```python
from build123d import *
from build123d.topology import SkipClean

# Parameters (mm, degrees)
SKETCH1_W           = 52.3
SKETCH1_H           = 52.3
SKETCH1_R           = 11.5
SKETCH1_R_2         = 1.75
BOSS_EXTRUDE1_DEPTH = 3
SKETCH2_W           = 52.3
SKETCH2_H           = 5
BOSS_EXTRUDE2_DEPTH = 40
SKETCH3_W           = 3
SKETCH3_H           = 5
CUT_EXTRUDE1_DEPTH  = 71.845695
BOSS_EXTRUDE3_DEPTH = 4.9
FILLET1_R           = 5
FILLET2_R           = 2
SKETCH5_W           = 10
SKETCH5_H           = 7
SKETCH5_R           = 1.3
BOSS_EXTRUDE4_DEPTH = 5
SKETCH6_W           = 7
SKETCH6_H           = 10
SKETCH6_R           = 1.35
BOSS_EXTRUDE5_DEPTH = 5
FILLET3_R           = 3
FILLET4_R           = 3
SKETCH7_R           = 3.3734375
BOSS_EXTRUDE6_DEPTH = 25.4
FILLET5_R           = 2
CUT_EXTRUDE2_DEPTH  = 85.05422357
FILLET6_START       = -26.15
FILLET6_DEPTH       = 7.129662431
FILLET6_START_2     = -20.042964894
FILLET6_2_DEPTH     = 4.85752147
FILLET6_START_3     = -16.0065624
FILLET6_3_DEPTH     = 2.695573852
FILLET6_4_DEPTH     = 1.974476163
FILLET6_5_DEPTH     = 1.685079156
FILLET6_START_4     = 2.9999999
FILLET6_6_DEPTH     = 22.4000001
FILLET6_START_5     = 5.780256625
FILLET6_7_DEPTH     = 0.960746932


with BuildPart() as part:
    # Sketch1 → Boss-Extrude1 (new body)
    with BuildSketch(Plane.XY):
        Rectangle(SKETCH1_W, SKETCH1_H)
        Circle(SKETCH1_R, mode=Mode.SUBTRACT)
        with Locations((-15.5, 15.5)):
            Circle(SKETCH1_R_2, mode=Mode.SUBTRACT)
        with Locations((15.5, 15.5)):
            Circle(SKETCH1_R_2, mode=Mode.SUBTRACT)
        with Locations((-15.5, -15.5)):
            Circle(SKETCH1_R_2, mode=Mode.SUBTRACT)
        with Locations((15.5, -15.5)):
            Circle(SKETCH1_R_2, mode=Mode.SUBTRACT)
    extrude(amount=BOSS_EXTRUDE1_DEPTH)

    # Sketch2 → Boss-Extrude2 (add)
    with BuildSketch(Plane(origin=(0, 0, 0), x_dir=(-1, 0, 0), z_dir=(0, 0, -1))):
        with Locations((0, -23.65)):
            Rectangle(SKETCH2_W, SKETCH2_H)
    extrude(amount=BOSS_EXTRUDE2_DEPTH)

    # Sketch3 → Cut-Extrude1 (cut, through all)
    with BuildSketch(Plane(origin=(26.15, 0, 0), x_dir=(0, 0, -1), z_dir=(1, 0, 0))):
        with Locations((-1.5, 23.65)):
            Rectangle(SKETCH3_W, SKETCH3_H)
    extrude(amount=-CUT_EXTRUDE1_DEPTH, mode=Mode.SUBTRACT)

    # Sketch4 → Boss-Extrude3 (add)
    with BuildSketch(Plane(origin=(26.15, 0, 0), x_dir=(0, 0, -1), z_dir=(1, 0, 0))):
        Polygon((0, 16.15), (25, -21.15), (20.184652233, -21.15), (0, 8.965501131), align=None)
    boss_extrude3 = extrude(amount=-BOSS_EXTRUDE3_DEPTH)

    # Mirror1: Boss-Extrude3 across plane
    add(boss_extrude3.mirror(Plane(origin=(0, 0, 0), x_dir=(0, 0, 1), z_dir=(1, 0, 0))))

    # Fillet1
    fillet1_edges = [part.edges().sort_by_distance(p)[0] for p in [
        (-26.15, -23.65, -40),
        (26.15, -23.65, -40),
        (-26.15, 21.15, 1.5),
        (26.15, 21.15, 1.5),
    ]]
    fillet(fillet1_edges, radius=FILLET1_R)

    # Fillet2
    fillet2_edges = [part.edges().sort_by_distance(p)[0] for p in [
        (23.7, 8.965501131, 0),
        (23.7, 16.15, 0),
        (23.7, -21.15, -25),
        (23.7, -21.15, -20.184652233),
        (-23.7, 16.15, 0),
        (-23.7, 8.965501131, 0),
        (-23.7, -21.15, -20.184652233),
        (-23.7, -21.15, -25),
    ]]
    fillet(fillet2_edges, radius=FILLET2_R)

    # Sketch5 → Boss-Extrude4 (add)
    with BuildSketch(Plane(origin=(0, -26.15, 0), x_dir=(1, 0, 0), z_dir=(0, 1, 0))):
        with Locations((-31.15, 0.5)):
            Rectangle(SKETCH5_W, SKETCH5_H)
        with Locations((-32.15, 0.5)):
            Circle(SKETCH5_R, mode=Mode.SUBTRACT)
    boss_extrude4 = extrude(amount=BOSS_EXTRUDE4_DEPTH)

    # Mirror2: Boss-Extrude4 across plane
    add(boss_extrude4.mirror(Plane(origin=(0, 0, 0), x_dir=(0, 0, 1), z_dir=(1, 0, 0))))

    # Sketch6 → Boss-Extrude5 (add)
    with BuildSketch(Plane.XZ.offset(26.15)):
        with Locations((0, -45)):
            Rectangle(SKETCH6_W, SKETCH6_H)
        with Locations(Location((0, -46, 0), (0, 0, 270))):
            Circle(SKETCH6_R, mode=Mode.SUBTRACT)
    extrude(amount=-BOSS_EXTRUDE5_DEPTH)

    # Fillet3
    fillet3_edges = [part.edges().sort_by_distance(p)[0] for p in [
        (-26.15, -23.65, -4),
        (-36.15, -23.65, -4),
        (-36.15, -23.65, 3),
        (36.15, -23.65, -4),
        (36.15, -23.65, 3),
        (26.15, -23.65, -4),
    ]]
    fillet(fillet3_edges, radius=FILLET3_R)

    # Fillet4
    fillet4_edges = [part.edges().sort_by_distance(p)[0] for p in [
        (3.5, -23.65, -50),
        (3.5, -23.65, -40),
        (-3.5, -23.65, -40),
        (-3.5, -23.65, -50),
    ]]
    fillet(fillet4_edges, radius=FILLET4_R)

    # Sketch7 → Boss-Extrude6 (add)
    with BuildSketch(Plane.XY.offset(3)):
        with BuildLine():
            Line((-26.15, 0), (-26.15, -26.15))
            Line((-26.15, -26.15), (-15.185443524, -26.15))
            ThreePointArc((-15.185443524, -26.15), (-20.234553545, -15.731999999), (-15.185443524, -5.313999997))
            ThreePointArc((-15.185443524, -5.313999997), (-16.427394993, 6.092210081), (-26.15, 0))
        make_face()
        with Locations((-19.38, 0)):
            Circle(SKETCH7_R, mode=Mode.SUBTRACT)
    extrude(amount=BOSS_EXTRUDE6_DEPTH)

    # Fillet5
    fillet5_edges = [part.edges().sort_by_distance(p)[0] for p in [
        (-15.185443524, -26.15, 15.7),
    ]]
    fillet(fillet5_edges, radius=FILLET5_R)

    # Sketch8 → Cut-Extrude2 (cut, through all)
    with BuildSketch(Plane.ZY.offset(26.15)):
        Polygon((8.005079096, -3), (25.4, -3), (25.4, -20.908550458), align=None)
        Polygon((5.347073795, -22.477794478), (23.248044349, -22.998786539), (5.853123446, -5.090236082), align=None)
    extrude(amount=-CUT_EXTRUDE2_DEPTH, mode=Mode.SUBTRACT)

    # Fillet6: read off the stored shape, not the designer's step
    # Fillet6 outline → Fillet6 (add)
    with BuildSketch(Plane.YZ.offset(FILLET6_START)):
        with BuildLine():
            ThreePointArc((-3, 12.735879268), (-4.221212944, 10.893736299), (-6.393490721, 11.301242168))
            Line((-6.393490721, 11.301242168), (-3, 8.005079096))
            Line((-3, 8.005079096), (-3, 12.735879268))
        make_face()
        with BuildLine():
            Line((-20.908550458, 25.4), (-17.372496907, 21.965362899))
            ThreePointArc((-17.372496907, 21.965362899), (-17.832283581, 24.151906177), (-15.979006186, 25.4))
            Line((-15.979006186, 25.4), (-20.908550458, 25.4))
        make_face()
        with BuildLine():
            ThreePointArc((-5, 25.4), (-3.585786438, 24.814213562), (-3, 23.4))
            Line((-3, 23.4), (-3, 25.4))
            Line((-3, 25.4), (-5, 25.4))
        make_face()
        with BuildLine():
            ThreePointArc((-22.855377198, 18.320586538), (-21.661726823, 20.209388823), (-19.462732989, 19.813407249))
            Line((-19.462732989, 19.813407249), (-22.998786539, 23.248044349))
            Line((-22.998786539, 23.248044349), (-22.855377198, 18.320586538))
        make_face()
        with BuildLine():
            Line((-5.090236082, 5.853123446), (-8.483726803, 9.149286517))
            ThreePointArc((-8.483726803, 9.149286517), (-8.013197931, 6.989783251), (-9.819033913, 5.715495928))
            Line((-9.819033913, 5.715495928), (-5.090236082, 5.853123446))
        make_face()
        with BuildLine():
            ThreePointArc((-20.47864099, 5.405257406), (-21.909297563, 5.94965388), (-22.535978089, 7.346227283))
            Line((-22.535978089, 7.346227283), (-22.477794478, 5.347073795))
            Line((-22.477794478, 5.347073795), (-20.47864099, 5.405257406))
        make_face()
    extrude(amount=FILLET6_DEPTH)

    # Fillet6 2 outline → Fillet6 2 (add)
    with BuildSketch(Plane.YZ.offset(FILLET6_START_2)):
        with BuildLine():
            ThreePointArc((-3, 12.735879268), (-4.221212944, 10.893736299), (-6.393490721, 11.301242168))
            Line((-6.393490721, 11.301242168), (-3, 8.005079096))
            Line((-3, 8.005079096), (-3, 12.735879268))
        make_face()
        with BuildLine():
            ThreePointArc((-5, 25.4), (-3.585786438, 24.814213562), (-3, 23.4))
            Line((-3, 23.4), (-3, 25.4))
            Line((-3, 25.4), (-5, 25.4))
        make_face()
        with BuildLine():
            Line((-5.090236082, 5.853123446), (-8.483726803, 9.149286517))
            ThreePointArc((-8.483726803, 9.149286517), (-8.013197931, 6.989783251), (-9.819033913, 5.715495928))
            Line((-9.819033913, 5.715495928), (-5.090236082, 5.853123446))
        make_face()
    extrude(amount=FILLET6_2_DEPTH)

    # Fillet6 3 outline → Fillet6 3 (add)
    with BuildSketch(Plane.YZ.offset(FILLET6_START_3)):
        with BuildLine():
            ThreePointArc((-3, 12.735879268), (-4.221212944, 10.893736299), (-6.393490721, 11.301242168))
            Line((-6.393490721, 11.301242168), (-3, 8.005079096))
            Line((-3, 8.005079096), (-3, 12.735879268))
        make_face()
        with BuildLine():
            ThreePointArc((-5, 25.4), (-3.585786438, 24.814213562), (-3, 23.4))
            Line((-3, 23.4), (-3, 25.4))
            Line((-3, 25.4), (-5, 25.4))
        make_face()
    extrude(amount=FILLET6_3_DEPTH)

    # Fillet6 4 outline → Fillet6 4 (add)
    with BuildSketch(Plane.YZ.offset(FILLET6_START_2)):
        with BuildLine():
            ThreePointArc((-22.855377198, 18.320586538), (-21.661726823, 20.209388823), (-19.462732989, 19.813407249))
            Line((-19.462732989, 19.813407249), (-22.998786539, 23.248044349))
            Line((-22.998786539, 23.248044349), (-22.855377198, 18.320586538))
        make_face()
    extrude(amount=FILLET6_4_DEPTH)

    # Fillet6 5 outline → Fillet6 5 (add)
    with BuildSketch(Plane.YZ.offset(FILLET6_START_2)):
        with BuildLine():
            ThreePointArc((-20.47864099, 5.405257406), (-21.909297563, 5.94965388), (-22.535978089, 7.346227283))
            Line((-22.535978089, 7.346227283), (-22.477794478, 5.347073795))
            Line((-22.477794478, 5.347073795), (-20.47864099, 5.405257406))
        make_face()
    extrude(amount=FILLET6_5_DEPTH)

    # Fillet6 6 outline → Fillet6 6 (cut)
    with SkipClean():  # the faces are left unmerged after this step: merging them gives an invalid solid
        with BuildSketch(Plane.XY.offset(FILLET6_START_4)):
            with BuildLine():
                Line((-18.03638138, -23.047623669), (-17.407246032, -24))
                Line((-17.407246032, -24), (-13.310988548, -24))
                Line((-13.310988548, -24), (-13.310988548, -3))
                ThreePointArc((-13.310988548, -3), (-14.11940539, -4.261343022), (-15.185443524, -5.313999997))
                ThreePointArc((-15.185443524, -5.313999997), (-20.066293198, -13.625309136), (-18.03638138, -23.047623669))
            make_face()
            with BuildLine():
                Line((-17.837249026, -3), (-20.922750974, -3))
                ThreePointArc((-20.922750974, -3), (-19.38, -3.3734375), (-17.837249026, -3))
            make_face()
        extrude(amount=FILLET6_6_DEPTH, mode=Mode.SUBTRACT)

    # Fillet6 7 outline → Fillet6 7 (add)
    with BuildSketch(Plane.XY.offset(FILLET6_START_5)):
        with BuildLine():
            Line((-15.185443424, -1), (-15.185443524, -5.313999997))
            ThreePointArc((-15.185443524, -5.313999997), (-13.523185641, -3.395677481), (-12.68426255, -1))
            Line((-12.68426255, -1), (-15.185443424, -1))
        make_face()
    extrude(amount=FILLET6_7_DEPTH)


solid = part.part
```
Build history of the part. All positions in model axes, mm. A direction names the side the tool comes from. Coordinates: 2 decimals unless noted, no trailing zeros. Write each loop counter-clockwise with the first axis right and the second up, starting at its lowest first coordinate (ties: lowest second). Pieces come first, ordered by that corner, then holes.
1. Drill centre lines: probe 1 along Y at (x, z) = (15.5, 1.95); probe 2 along Z at (x, y) = (-23, -15); probe 3 along X at (y, z) = (0, 10.25). Where is each one in solid material? Low to high.
Answer block:
probe 1: y = -26.15 to -17.25, -13.75 to 13.75, 17.25 to 21.15
probe 2: z = -20.88 to -16.06, 0 to 5.56, 15.48 to 19.66, 25.4 to 28.4
probe 3: x = -26.15 to -22.75, -16.01 to -12.61
2. Band-saw the part on C-C, the plane x = 25. Give the cut face in (y, z), and give its area (3 significant figures).
Answer block:
outline: (-26.15, -38.19) - (-21.15, -38.19) - (-21.15, -26.07) arc R2 cw to (-20.26, -24.41) - (15.64, -0.34) arc R2 cw to (16.76, 0) - (19.34, 0) - (19.34, 3) - (-26.15, 3) - close; hole (-21.15, -16.44) arc R2 ccw to (-18.04, -18.1) - (3.5, -3.66) arc R2 ccw to (2.39, 0) - (-21.15, 0) - close
area: 501 mm2
3. Band-saw the part on D-D, the plane z = 14.5. Give the cut face in (x, y), and give its area (3 significant figures).
Answer block:
outline: (-26.15, -26.15) - (-19.71, -26.15) arc R2 ccw to (-18.04, -23.05) arc R13.27 cw to (-18.23, -22.74) - (-26.15, -22.74) - close; (-26.15, -13.99) - (-20.12, -13.99) arc R13.27 cw to (-18.78, -9.69) - (-26.15, -9.69) - close; (-26.15, -3) - (-20.92, -3) arc R3.37 cw (long way) to (-17.84, -3) - (-13.31, -3) arc R6.77 ccw (long way) to (-26.15, 0) - close
area: 133 mm2
4. Drop flat-ended pins along their axis: pin 1 (1.5 mm diameter, centred on y = -20, z = -12, fed in from +X); pin 2 (8 mm diameter, centred on y = -19, z = -10.5, fed in from -X); pin 3 (2.5 mm diameter, centred on x = 14, y = -22.5, fed in from -Z); pin 4 (4 mm diameter, centred on x = -30.5, y = -23, fed in from +Z). Give the stop position or say it passes through.
Answer block:
pin 1: passes through
pin 2: stops at x = -26.15
pin 3: stops at z = -40
pin 4: stops at z = 3
5. 3-axis set-ups, long thin cutter, end or side, ignore diameter. For faces 4 (the flat face through (-31, -24, -4)), 5 (the flat face through (-23.068, -14.05, 14.556)), 6 (the flat face through (-12, 0, 0)), 7 (the flat face through (21.25, -4, -11)), 8 (the cylindrical face through (-17.958, -25.124, 15.878)): which of +Z, -Z, +X, -X, +Y, -Y reach the whole face in a straight line?
Answer block:
face 4: -Z, -X, +Y, -Y
face 5: +X, -X
face 6: none
face 7: -Z, +Y
face 8: +Z, +X
6. Pull direction X, two halves, no side cores. Call faces 1 (the cylindrical face through (24.72, -23.62, -38.5)), 2 (the flat face through (0, 21.15, 2)), 3 (the cylindrical face through (-30.91, -23.68, -0.89)): released by +X, released by -X, zero draft, split by the parting line, or undercut.
Answer block:
face 1: released by +X
face 2: zero draft
face 3: undercut
7. Band-saw the part on B-B, the plane x = -9.5. Give the cut face in (y, z), and give its area (3 significant figures).
Answer block:
outline: (-26.15, -40) - (-21.15, -40) - (-21.15, 0) - (-6.48, 0) - (-6.48, 3) - (-26.15, 3) - close; (6.48, 0) - (21.15, 0) - (21.15, 3) - (6.48, 3) - close
area: 303 mm2
8. Band-saw the part on A-A, the plane z = -46. Give the cut face in (x, y), and give its area (3 significant figures).
Answer block:
outline: (-3.5, -26.15) - (-1.35, -26.15) - (-1.35, -21.15) - (-3.5, -21.15) - close; (1.35, -26.15) - (3.5, -26.15) - (3.5, -21.15) - (1.35, -21.15) - close
area: 21.5 mm2
